Can you work these out from the model? Positions are in its coordinate system, mm. Face numbers are marked on the shaded views. A direction names the side the tool comes from. Give positions to 0.01 mm unless a question says otherwise; leave off trailing zeros. Order: outer loops, then holes, each group sorted by start corner. A loop starts at its lowest first (then second) coordinate and runs counter-clockwise, first axis right, second up. Notation, with made-up numbers: (42, 16) - (54, 16) arc R24 cw to (54, 48) - close; hole circle Ø4 at (-19, -29). An arc over 180 degrees is marked (long way). Answer as a JSON object with one key per item and string values.
```python
from build123d import *

# Parameters (mm, degrees)
SKETCH4_R               = 17.5
BOSS_EXTRUDE1_DEPTH     = 2
BOSS_EXTRUDE2_DEPTH     = 4
BOSS_EXTRUDE3_DEPTH     = 10
SKETCH6_R               = 2.1
CUT_EXTRUDE1_DEPTH      = 3
CUT_EXTRUDE1_DEPTH_BACK = 13


with BuildPart() as part:
    # Sketch4 → Boss-Extrude1 (new body)
    with BuildSketch(Plane(origin=(0, 0, 0), x_dir=(1, 0, 0), z_dir=(0, 1, 0))):
        Circle(SKETCH4_R)
    extrude(amount=BOSS_EXTRUDE1_DEPTH)

    # Sketch1 → Boss-Extrude2 (add)
    with BuildSketch(Plane(origin=(0, 0, 0), x_dir=(1, 0, 0), z_dir=(0, 1, 0))):
        with BuildLine():
            Line((-8.26, 15), (8.26, 15))
            ThreePointArc((8.26, 15), (0, 6.74), (-8.26, 15))
        make_face()
        with BuildLine():
            Line((15, 8.26), (15, -8.26))
            ThreePointArc((15, -8.26), (6.74, 0), (15, 8.26))
        make_face()
        with BuildLine():
            Line((8.26, -15), (-8.26, -15))
            ThreePointArc((-8.26, -15), (0, -6.74), (8.26, -15))
        make_face()
        with BuildLine():
            Line((-15, -8.26), (-15, 8.26))
            ThreePointArc((-15, 8.26), (-6.74, 0), (-15, -8.26))
        make_face()
    extrude(amount=BOSS_EXTRUDE2_DEPTH)

    # Sketch5 → Boss-Extrude3 (add)
    with BuildSketch(Plane.XZ):
        Polygon((-6.619767116, 2.044182802), (-5.080197795, -4.710795089), (1.539569322, -6.754977891), (6.619767116, -2.044182802), (5.080197795, 4.710795089), (-1.539569322, 6.754977891), align=None)
    extrude(amount=BOSS_EXTRUDE3_DEPTH)

    # Sketch6 → Cut-Extrude1 (cut, two sides)
    with BuildSketch(Plane(origin=(0, 2, 0), x_dir=(1, 0, 0), z_dir=(0, 1, 0))) as cut_extrude1_sk:
        Circle(SKETCH6_R)
    extrude(amount=CUT_EXTRUDE1_DEPTH, mode=Mode.SUBTRACT)
    extrude(cut_extrude1_sk.sketch, amount=-CUT_EXTRUDE1_DEPTH_BACK, mode=Mode.SUBTRACT)


solid = part.part
```
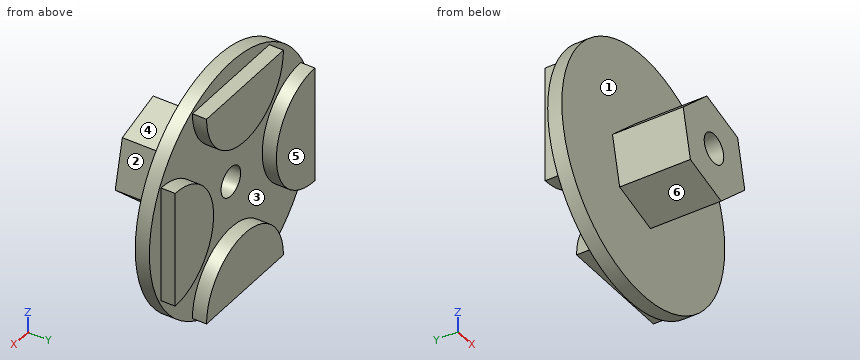
Q1. I'm going to push flat-ended pins straight in: pin 1 Ø1 at (y, z) = (3, 0) entering from -X; pin 2 Ø5 at (x, y) = (4, -7.5) entering from +Z; pin 3 Ø3 at (y, z) = (0, 10.5) entering from +X; pin 4 Ø4 at (x, z) = (0, 0) entering from -Y. Where does each tip first touch, or does it pass through?
Recorded:
{"pin 1": "stops at x = -15", "pin 2": "stops at z = 5.82", "pin 3": "stops at x = 15.01", "pin 4": "passes through"}
Q2. We'd pull the mould along Z, two halves only. Please class the marked faces 1, 2 and 3: released by +Z, released by -Z, zero draft, split by the parting line, or undercut.
Recorded:
{"face 1": "zero draft", "face 2": "released by +Z", "face 3": "undercut"}
Q3. If we section it at D-D, the plane x = -13: Please give me the cut outline in (y, z).
Recorded:
{"outline": "(0, -11.72) - (2, -11.72) - (2, -8.01) - (4, -8.01) - (4, 8.01) - (2, 8.01) - (2, 11.72) - (0, 11.72) - close"}
Q4. If we section it at C-C, the plane x = 0: Please give me the cut outline in (y, z).
Recorded:
{"outline": "(-10, -6.28) - (0, -6.28) - (0, -17.5) - (2, -17.5) - (2, -15) - (4, -15) - (4, -6.74) - (2, -6.74) - (2, -2.1) - (-10, -2.1) - close; (-10, 2.1) - (2, 2.1) - (2, 6.74) - (4, 6.74) - (4, 15) - (2, 15) - (2, 17.5) - (0, 17.5) - (0, 6.28) - (-10, 6.28) - close"}
Q5. Which directions (+Z, -Z, +X, -X, +Y, -Y) give clear straight access to the entire face, cutting with the end or side of a thin tool? Please do the marked faces 4, 5 and 6.
Recorded:
{"face 4": "+Z, +X, -Y", "face 5": "+Z, -Z, +X, -X, +Y", "face 6": "-Z, -X, -Y"}
Q6. I need wall thicknesses on L1, parallel to Y at x = -10, z = 10; L2, parallel to Y at x = -3.5, z = 11; L3, parallel to Z at x = -6, y = 3. Which ranges of each line are inside material? Lowest first, please.
Recorded:
{"L1": "y = 0 to 2", "L2": "y = 0 to 4", "L3": "z = -15 to -9.32, 9.32 to 15"}
Q7. If we section it at B-B, the plane z = 1: Please give me the cut outline in (x, y).
Recorded:
{"outline": "(-17.47, 0) - (-6.38, 0) - (-6.38, -10) - (-1.85, -10) - (-1.85, 2) - (-6.8, 2) - (-6.8, 4) - (-15, 4) - (-15, 2) - (-17.47, 2) - close; (1.85, -10) - (5.93, -10) - (5.93, 0) - (17.47, 0) - (17.47, 2) - (15, 2) - (15, 4) - (6.8, 4) - (6.8, 2) - (1.85, 2) - close"}
Q8. If we section it at A-A, the plane y = -9: Please give me the cut outline in (x, z), then the cut area to 3 significant figures.
Recorded:
{"outline": "(-6.62, 2.04) - (-5.08, -4.71) - (1.54, -6.75) - (6.62, -2.04) - (5.08, 4.71) - (-1.54, 6.75) - close; hole circle Ø4.2 at (0, 0)", "area": "111 mm^2"}
